Design review of the part built by this model. Coordinates are the model's own, in mm. Face numbers are marked on the shaded views. Coordinates: 2 decimals unless noted, no trailing zeros. Loops run counter-clockwise (first coordinate to the right, second up) from the corner with the lowest first, then second, coordinate; pieces in that order, holes last. Notation, with made-up numbers: M -36,-32.5 L 2,-32.5 A34 ccw 2,-1.5 Z; hole C -8.5,30 d5. An arc over 180 degrees is marked long. Answer as a JSON object with one key per item and string values. Group by question number.
1. Consider section C-C (y = -34). State the section outline as (x, z) points.
2. Consider section D-D (z = 18). State the section outline as (x, y) points.
3. Consider section B-B (x = 4). State the section outline as (y, z) points, then the cut area to 3 significant figures.
4. Consider section A-A (x = -86.5). State the section outline as (y, z) points, then the cut area to 3 significant figures.
5. To check wall thickness, follow probe 1 along Y at (x, z) = (80, 48.35); probe 2 along Y at (x, z) = (46.3, 48.15); probe 3 along Z at (x, y) = (57.5, 5.5). State the ranges of each line that lie inside material, in increasing order.
6. Insertion check: pin 1 (2.5 mm diameter, centred on x = -16.07, y = 4.13, fed in from -Z); pin 2 (2 mm diameter, centred on x = -74, z = 32.5, fed in from -Y); pin 3 (6 mm diameter, centred on y = -33, z = 15.5, fed in from +X); pin 4 (2.5 mm diameter, centred on y = -46.5, z = 47.5, fed in from +X). Each pin has a flat end and moves straight along its axis. Give the tip position at first contact, or say it passes through.
7. Draft analysis for pull direction X (two halves, no side actions). For the marked faces 1, 2, 3 and 4, state which applies: +X half, -X half, draft (parallel to the pull), parting line (faces both ways), or undercut.
from build123d import *

# Parameters (mm, degrees)
ESQUISSE1_R              = 105
BOSS_EXTRU_1_DEPTH       = 50
COQUE1_T                 = -5
ESQUISSE3_R              = 25
ESQUISSE3_R_2            = 1.5
ENL_V_MAT_EXTRU_1_DEPTH  = 10
ENL_V_MAT_EXTRU_2_DEPTH  = 156.161206492
ENL_V_MAT_EXTRU_3_DEPTH  = 45
ESQUISSE7_R              = 1.5
ENL_V_MAT_EXTRU_4_DEPTH  = 156.161206492
ESQUISSE8_W              = 11
ESQUISSE8_H              = 31.895350387
ENL_V_MAT_EXTRU_5_DEPTH  = 5
ESQUISSE9_R              = 15.5
ENL_V_MAT_EXTRU_7_DEPTH  = 156.161206492
BALAYAGE1_PROFILE_R      = 1.5
BOSS_EXTRU_2_START       = 1
BOSS_EXTRU_2_DEPTH       = 1
BALAYAGE2_PROFILE_R      = 1.5
BOSS_EXTRU_3_START       = 2
BOSS_EXTRU_3_DEPTH       = 2
ESQUISSE30_R             = 1.5
BOSS_EXTRU_4_DEPTH       = 5
ESQUISSE31_R             = 12
ENL_V_MAT_EXTRU_8_DEPTH  = 5
ESQUISSE32_W             = 5.713355649
ESQUISSE32_H             = 13.88652285
ENL_V_MAT_EXTRU_10_DEPTH = 352.816395688


with BuildPart() as part:
    # Esquisse1 → Boss.-Extru.1 (new body)
    with BuildSketch(Plane.XY):
        Circle(ESQUISSE1_R)
    extrude(amount=BOSS_EXTRU_1_DEPTH)

    # Coque1
    coque1_openings = [part.faces().sort_by_distance(p)[0] for p in [
        (0, 0, 0),
    ]]
    offset(amount=COQUE1_T, openings=coque1_openings, kind=Kind.INTERSECTION)

    # Esquisse3 → Enlèv. mat.-Extru.1 (cut)
    with BuildSketch(Plane(origin=(0, 0, 45), x_dir=(-1, 0, 0), z_dir=(0, 0, -1))):
        with Locations((-3.8, -24.557615642)):
            Circle(ESQUISSE3_R)
        with Locations((-23.669465397, 4.134521322)):
            Circle(ESQUISSE3_R_2)
        with Locations((16.069465397, 4.134521322)):
            Circle(ESQUISSE3_R_2)
        with Locations((31.7, -51.557615642)):
            Circle(ESQUISSE3_R_2)
    extrude(amount=-ENL_V_MAT_EXTRU_1_DEPTH, mode=Mode.SUBTRACT)

    # Esquisse5 → Enlèv. mat.-Extru.2 (cut, through all)
    with BuildSketch(Plane(origin=(0, 0, 45), x_dir=(-1, 0, 0), z_dir=(0, 0, -1))):
        with BuildLine():
            Line((-42.388918531, 10.472597699), (35.07440103, 10.472597699))
            ThreePointArc((35.07440103, 10.472597699), (37.195721374, 11.351277356), (38.07440103, 13.472597699))
            Line((38.07440103, 13.472597699), (38.07440103, 45.806945365))
            ThreePointArc((38.07440103, 45.806945365), (37.195721374, 47.928265708), (35.07440103, 48.806945365))
            Line((35.07440103, 48.806945365), (-42.388918531, 48.806945365))
            ThreePointArc((-42.388918531, 48.806945365), (-44.510238875, 47.928265708), (-45.388918531, 45.806945365))
            Line((-45.388918531, 45.806945365), (-45.388918531, 13.472597699))
            ThreePointArc((-45.388918531, 13.472597699), (-44.510238875, 11.351277356), (-42.388918531, 10.472597699))
        make_face()
    extrude(amount=-ENL_V_MAT_EXTRU_2_DEPTH, mode=Mode.SUBTRACT)

    # Esquisse6 → Enlèv. mat.-Extru.3 (cut)
    with BuildSketch(Plane(origin=(0, 0, 0), x_dir=(-1, 0, 0), z_dir=(0, 0, -1))):
        with BuildLine():
            Line((-78.81072608, -69.38205427), (78.81072608, -69.38205427))
            ThreePointArc((78.81072608, -69.38205427), (0, -105), (-78.81072608, -69.38205427))
        make_face()
    extrude(amount=-ENL_V_MAT_EXTRU_3_DEPTH, mode=Mode.SUBTRACT)

    # Esquisse7 → Enlèv. mat.-Extru.4 (cut, through all)
    with BuildSketch(Plane(origin=(0, 0, 45), x_dir=(-1, 0, 0), z_dir=(0, 0, -1))):
        with Locations((52.614229855, 48.990085475)):
            Circle(ESQUISSE7_R)
        with Locations((52.614229855, 11.990085475)):
            Circle(ESQUISSE7_R)
        with Locations((46.3, -26.057615642)):
            Circle(ESQUISSE7_R)
        with Locations((46.3, -53.057615642)):
            Circle(ESQUISSE7_R)
        with Locations((-46.3, -26.062213408)):
            Circle(ESQUISSE7_R)
        with Locations((-46.3, -53.062213408)):
            Circle(ESQUISSE7_R)
    extrude(amount=-ENL_V_MAT_EXTRU_4_DEPTH, mode=Mode.SUBTRACT)

    # Esquisse8 → Enlèv. mat.-Extru.5 (cut)
    with BuildSketch(Plane(origin=(0, 0, 45), x_dir=(-1, 0, 0), z_dir=(0, 0, -1))):
        with Locations((-75.3, -39.589403314)):
            Rectangle(ESQUISSE8_W, ESQUISSE8_H)
        with Locations((75.3, -39.589403314)):
            Rectangle(ESQUISSE8_W, ESQUISSE8_H)
    extrude(amount=-ENL_V_MAT_EXTRU_5_DEPTH, mode=Mode.SUBTRACT)

    # Esquisse9 → Enlèv. mat.-Extru.7 (cut, through all)
    with BuildSketch(Plane(origin=(0, 0, 45), x_dir=(-1, 0, 0), z_dir=(0, 0, -1))):
        with Locations((34.681880454, 70.440085475)):
            Circle(ESQUISSE9_R)
        with Locations((-34.681880454, 70.440085475)):
            Circle(ESQUISSE9_R)
    extrude(amount=-ENL_V_MAT_EXTRU_7_DEPTH, mode=Mode.SUBTRACT)

    # Balayage1: sweep along a path in Esquisse10
    with BuildLine(Plane(origin=(-9.681880454, 0.440085475, 22), x_dir=(-1, 0, 0), z_dir=(0, 0, -1))) as balayage1_path:
        Line((-43.221417057, 88.965628134), (-42.925873334, 93.872357698))
    # Balayage1 profile (on start of the path) → Balayage1 (sweep)
    with BuildSketch(Plane(origin=(33.539536603, 89.405713609, 22), x_dir=(0.9981909544337458, 0.060123360573471965, 0), z_dir=(-0.060123360573471965, 0.9981909544337458, 0))):
        Circle(BALAYAGE1_PROFILE_R)
    balayage1 = sweep(path=balayage1_path.line)

    # Esquisse19 → Boss.-Extru.2 (add)
    with BuildSketch(Plane(origin=(-5.53995205, 91.976396052, 0), x_dir=(0.998190954433746, 0.06012336057346903, 0), z_dir=(-0.06012336057346903, 0.998190954433746, 0)).offset(BOSS_EXTRU_2_START)):
        with BuildLine():
            Line((38.85423401, -23.5), (38.85423401, -20.5))
            ThreePointArc((38.85423401, -20.5), (37.35423401, -22), (38.85423401, -23.5))
        make_face()
    boss_extru_2 = extrude(amount=-BOSS_EXTRU_2_DEPTH)

    # Balayage2: sweep along a path in Esquisse20
    with BuildLine(Plane(origin=(-9.681880454, 0.440085475, 22), x_dir=(-1, 0, 0), z_dir=(0, 0, -1))) as balayage2_path:
        Line((-73.311298587, 71.743577457), (-78.469516131, 72.142702967))
    # Balayage2 profile (on start of the path) → Balayage2 (sweep)
    with BuildSketch(Plane(origin=(63.629418133, 72.183662932, 22), x_dir=(-0.07714603625431019, 0.9970198037603109, 0), z_dir=(0.9970198037603109, 0.07714603625431019, 0))):
        Circle(BALAYAGE2_PROFILE_R)
    balayage2 = sweep(path=balayage2_path.line)

    # Esquisse27 → Boss.-Extru.3 (add)
    with BuildSketch(Plane(origin=(73.961032209, 5.722855705, 0), x_dir=(0, 0, -1), z_dir=(0.9970198037603113, 0.07714603625430425, 0)).offset(BOSS_EXTRU_3_START)):
        with BuildLine():
            Line((-20.5, 67.059784053), (-23.5, 67.059784053))
            ThreePointArc((-23.5, 67.059784053), (-22, 65.559784053), (-20.5, 67.059784053))
        make_face()
    boss_extru_3 = extrude(amount=-BOSS_EXTRU_3_DEPTH)

    # Symétrie1: Balayage1, Boss.-Extru.2, Balayage2, Boss.-Extru.3 across plane
    add(balayage1.mirror(Plane(origin=(0, 0, 0), x_dir=(0, 0, 1), z_dir=(1, 0, 0))))
    add(boss_extru_2.mirror(Plane(origin=(0, 0, 0), x_dir=(0, 0, 1), z_dir=(1, 0, 0))))
    add(balayage2.mirror(Plane(origin=(0, 0, 0), x_dir=(0, 0, 1), z_dir=(1, 0, 0))))
    add(boss_extru_3.mirror(Plane(origin=(0, 0, 0), x_dir=(0, 0, 1), z_dir=(1, 0, 0))))

    # Esquisse30 → Boss.-Extru.4 (add)
    with BuildSketch(Plane(origin=(0, 0, 0), x_dir=(-1, 0, 0), z_dir=(0, 0, -1))):
        with Locations(Location((0, 102.5, 0), (0, 0, 180))):
            Circle(ESQUISSE30_R)
        with Locations(Location((-72.478445072, 72.478445072, 0), (0, 0, 180))):
            Circle(ESQUISSE30_R)
        with Locations((72.478445072, 72.478445072)):
            Circle(ESQUISSE30_R)
    extrude(amount=BOSS_EXTRU_4_DEPTH)

    # Esquisse31 → Enlèv. mat.-Extru.8 (cut)
    with BuildSketch(Plane(origin=(0, 0, 45), x_dir=(-1, 0, 0), z_dir=(0, 0, -1))):
        with Locations((-80, 25)):
            Circle(ESQUISSE31_R)
        with Locations((80, 25)):
            Circle(ESQUISSE31_R)
    extrude(amount=-ENL_V_MAT_EXTRU_8_DEPTH, mode=Mode.SUBTRACT)

    # Esquisse32 → Enlèv. mat.-Extru.10 (cut, through all)
    with BuildSketch(Plane(origin=(91.985124309, -26.801506348, -210), x_dir=(0, 0, -1), z_dir=(0.9659258262890654, -0.25881904510253173, 0))):
        with Locations((-251.407492867, 19.659218808)):
            Rectangle(ESQUISSE32_W, ESQUISSE32_H)
    extrude(amount=ENL_V_MAT_EXTRU_10_DEPTH, mode=Mode.SUBTRACT)


solid = part.part
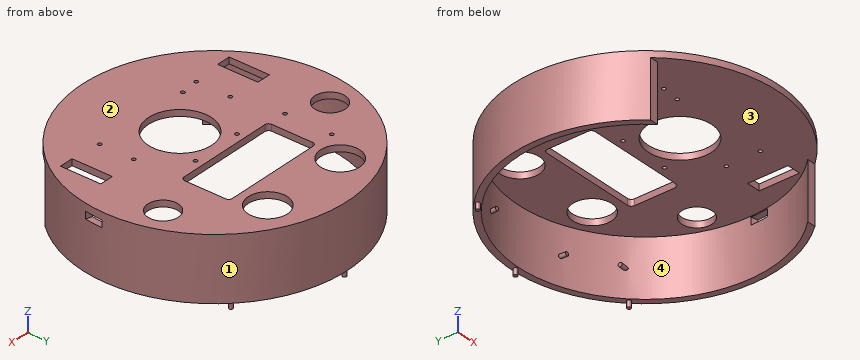
Findings below:
{
 "1": {"outline": "M -99.34,0 L -94.04,0 L -94.04,45 L -80.8,45 L -80.8,50 L -99.34,50 Z; M -69.8,45 L -19.35,45 L -19.35,50 L -69.8,50 Z; M 26.95,45 L 69.8,45 L 69.8,50 L 26.95,50 Z; M 80.8,45 L 94.04,45 L 94.04,0 L 99.34,0 L 99.34,50 L 80.8,50 Z"},
 "2": {"outline": "M -78.81,-69.38 L -72.01,-69.38 A100 cw long 72.01,-69.38 L 78.81,-69.38 A105 ccw long Z"},
 "3": {"outline": "M -104.92,45 L -49.56,45 L -49.56,50 L -104.92,50 Z; M 0.44,45 L 10.47,45 L 10.47,50 L 0.44,50 Z; M 48.81,45 L 99.92,45 L 99.92,0 L 104.92,0 L 104.92,50 L 48.81,50 Z", "area": "833 mm^2"},
 "4": {"outline": "M -59.52,0 L -50.18,0 L -50.18,45 L 14.91,45 L 14.91,50 L -59.52,50 Z; M 35.09,45 L 50.18,45 L 50.18,0 L 59.52,0 L 59.52,50 L 35.09,50 Z", "area": "1,340 mm^2"},
 "5": {"probe 1": "y = -68.01 to -55.54, -23.64 to 13, 37 to 68.01", "probe 2": "y = -94.24 to -54.56, -51.56 to -27.56, -24.56 to 60.18, 80.7 to 94.24", "probe 3": "z = 45 to 50"},
 "6": {"pin 1": "passes through", "pin 2": "stops at y = -69.38", "pin 3": "stops at x = 100.62", "pin 4": "stops at x = 94.75"},
 "7": {"face 1": "parting line", "face 2": "draft", "face 3": "undercut", "face 4": "undercut"}
}
